Design review of the part built by this model. Coordinates are the model's own, in mm. Face numbers are marked on the shaded views. A direction names the side the tool comes from. Coordinates: 2 decimals unless noted, no trailing zeros. Write each loop counter-clockwise with the first axis right and the second up, starting at its lowest first coordinate (ties: lowest second). Pieces come first, ordered by that corner, then holes. Notation, with made-up numbers: (-16.75, -24.5) -> (17.25, -24.5) arc R9 ccw to (17.25, -20.5) -> close; hole circle Ø8 at (1, -39.5). An arc over 180 degrees is marked (long way). Answer in a Markdown table with one row per item. Add a question column.
Item 1: Draft analysis for pull direction X (two halves, no side actions). For the marked faces 3, 4 and 5, state which applies: released by +X, released by -X, zero draft, split by the parting line, or undercut.
Item 2: Clearance check with flat-ended pins moving along their axes: P1, Ø2, axis at x = 15.5, z = -15.5, coming from the -Y side; P2, Ø3, axis at x = -15.5, z = -16.5, coming from the -Y side. State where each tip first meets the part, or that it passes through.
Item 3: Take a section at D-D, the plane x = 0. Write out the cut boundary in (y, z), and give its area (3 significant figures).
Item 4: Take a section at A-A, the plane z = 15.5. Write out the cut boundary in (x, y), and give its area (3 significant figures).
Item 5: Take a section at B-B, the plane y = 10. Write out the cut boundary in (x, z).
Item 6: For the marked faces 1 and 2, list the 3-axis set-ups (+Z, -Z, +X, -X, +Y, -Y) from which the entire face can be reached by the end or side of a thin tool; tool diameter is ignored.
Item 7: To check wall thickness, follow line 1 (X direction, y = 3.75, z = 15.5); line 2 (X direction, y = 18.3, z = -15.5); line 3 (X direction, y = 3.75, z = 0.5). State the ranges of each line that lie inside material, in increasing order.
Item 8: Take a section at C-C, the plane x = 15.5. Write out the cut boundary in (y, z), and give its area (3 significant figures).
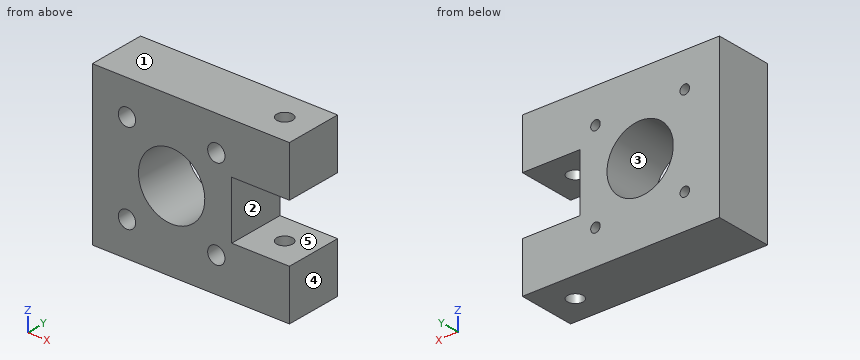
from build123d import *

# Parameters (mm, degrees)
SKETCH_1_R          = 1.65
SKETCH_1_R_2        = 11.5
EXTRUDE_1_DEPTH     = 20
SKETCH_6_W          = 17.5
SKETCH_6_H          = 20
EXTRUDE_2_DEPTH     = 20
SKETCH_7_R          = 3
CUT_EXTRUDE_1_DEPTH = 16
SKETCH_8_R          = 2.75
CUT_EXTRUDE_2_DEPTH = 72.370319461


with BuildPart() as part:
    # 草图1 → 凸台-拉伸1 (new body)
    with BuildSketch(Plane(origin=(0, 0, 0), x_dir=(1, 0, 0), z_dir=(0, 1, 0))):
        Polygon((20.85, 20.85), (20.85, 27.5), (-27.5, 27.5), (-27.5, -27.5), (20.85, -27.5), align=None)
        with Locations(Location((-15.5, 15.5, 0), (0, 0, 270))):
            Circle(SKETCH_1_R, mode=Mode.SUBTRACT)
        with Locations(Location((15.5, 15.5, 0), (0, 0, 270))):
            Circle(SKETCH_1_R, mode=Mode.SUBTRACT)
        with Locations(Location((15.5, -15.5, 0), (0, 0, 270))):
            Circle(SKETCH_1_R, mode=Mode.SUBTRACT)
        with Locations(Location((-15.5, -15.5, 0), (0, 0, 270))):
            Circle(SKETCH_1_R, mode=Mode.SUBTRACT)
        with Locations(Location((0, 0, 0), (0, 0, 270))):
            Circle(SKETCH_1_R_2, mode=Mode.SUBTRACT)
    extrude(amount=EXTRUDE_1_DEPTH)

    # 草图6 → 凸台-拉伸2 (add)
    with BuildSketch(Plane(origin=(20.85, 0, 0), x_dir=(0, 0, -1), z_dir=(1, 0, 0))):
        with Locations((18.75, 10)):
            Rectangle(SKETCH_6_W, SKETCH_6_H)
        with Locations((-18.75, 10)):
            Rectangle(SKETCH_6_W, SKETCH_6_H)
    extrude(amount=EXTRUDE_2_DEPTH)

    # 草图7 → 切除-拉伸1 (cut)
    with BuildSketch(Plane.XZ):
        with Locations(Location((-15.5, 15.5, 0), (0, 0, 270))):
            Circle(SKETCH_7_R)
        with Locations(Location((15.5, 15.5, 0), (0, 0, 270))):
            Circle(SKETCH_7_R)
        with Locations(Location((15.5, -15.5, 0), (0, 0, 270))):
            Circle(SKETCH_7_R)
        with Locations(Location((-15.5, -15.5, 0), (0, 0, 270))):
            Circle(SKETCH_7_R)
    extrude(amount=-CUT_EXTRUDE_1_DEPTH, mode=Mode.SUBTRACT)

    # 草图8 → 切除-拉伸2 (cut, through all)
    with BuildSketch(Plane(origin=(0, 0, -27.5), x_dir=(-1, 0, 0), z_dir=(0, 0, -1))):
        with Locations((-30.85, 10)):
            Circle(SKETCH_8_R)
    extrude(amount=-CUT_EXTRUDE_2_DEPTH, mode=Mode.SUBTRACT)


solid = part.part
Answers:
| question | item | result |
|---|---|---|
| 1 | face 3 | undercut |
| 1 | face 4 | released by +X |
| 1 | face 5 | zero draft |
| 2 | P1 | passes through |
| 2 | P2 | stops at y = 16 |
| 3 | outline | (0, -27.5) -> (20, -27.5) -> (20, -11.5) -> (0, -11.5) -> close; (0, 11.5) -> (20, 11.5) -> (20, 27.5) -> (0, 27.5) -> close |
| 3 | area | 640 mm^2 |
| 4 | outline | (-27.5, 0) -> (-18.5, 0) -> (-18.5, 16) -> (-17.15, 16) -> (-17.15, 20) -> (-27.5, 20) -> close; (-13.85, 16) -> (-12.5, 16) -> (-12.5, 0) -> (12.5, 0) -> (12.5, 16) -> (13.85, 16) -> (13.85, 20) -> (-13.85, 20) -> close; (17.15, 16) -> (18.5, 16) -> (18.5, 0) -> (40.85, 0) -> (40.85, 20) -> (17.15, 20) -> close; hole circle Ø5.5 at (30.85, 10) |
| 4 | area | 1,120 mm^2 |
| 5 | outline | (-27.5, -27.5) -> (28.1, -27.5) -> (28.1, -10) -> (20.85, -10) -> (20.85, 10) -> (28.1, 10) -> (28.1, 27.5) -> (-27.5, 27.5) -> close; (33.6, -27.5) -> (40.85, -27.5) -> (40.85, -10) -> (33.6, -10) -> close; (33.6, 10) -> (40.85, 10) -> (40.85, 27.5) -> (33.6, 27.5) -> close; hole circle Ø6 at (-15.5, -15.5); hole circle Ø6 at (-15.5, 15.5); hole circle Ø23 at (0, 0); hole circle Ø6 at (15.5, -15.5); hole circle Ø6 at (15.5, 15.5) |
| 6 | face 1 | +Z, +X, -X, +Y, -Y |
| 6 | face 2 | +X, +Y, -Y |
| 7 | line 1 | x = -27.5 to -18.5, -12.5 to 12.5, 18.5 to 40.85 |
| 7 | line 2 | x = -27.5 to -17.15, -13.85 to 13.85, 17.15 to 40.85 |
| 7 | line 3 | x = -27.5 to -11.49, 11.49 to 20.85 |
| 8 | outline | (0, -27.5) -> (20, -27.5) -> (20, -17.15) -> (16, -17.15) -> (16, -18.5) -> (0, -18.5) -> close; (0, -12.5) -> (16, -12.5) -> (16, -13.85) -> (20, -13.85) -> (20, 13.85) -> (16, 13.85) -> (16, 12.5) -> (0, 12.5) -> close; (0, 18.5) -> (16, 18.5) -> (16, 17.15) -> (20, 17.15) -> (20, 27.5) -> (0, 27.5) -> close |
| 8 | area | 882 mm^2 |
